The model under review builds one solid part; all positions refer to its coordinate system, in mm. A direction names the side the tool comes from. Coordinates: 2 decimals unless noted, no trailing zeros. Loops run counter-clockwise (first coordinate to the right, second up) from the corner with the lowest first, then second, coordinate; pieces in that order, holes last. Notation, with made-up numbers: M -39,13.5 L -30,13.5 A10 ccw -30,29.5 Z; hole C 13.5,83.25 d3. An arc over 180 degrees is marked long. Use one line per item in the form item = value.
Autodesk Inventor part; units mm, degrees
ref_plane "YZ Plane" through (0, 0, 0) normal (1, 0, 0) x (0, 1, 0)
ref_plane "XZ Plane" through (0, 0, 0) normal (0, 1, 0) x (-1, 0, 0)
ref_plane "XY Plane" through (0, 0, 0) normal (0, 0, 1) x (1, 0, 0)
sketch "Sketch1" plane through (0, 0, 0) normal (0, 0, 1) x (1, 0, 0)
  circle A0 centre (0, 0) radius 6.5
  dimension "d0" = 13
extrude "Extrusion1" add sketch "Sketch1" along normal blind 10
sketch "Sketch2" plane through (0, 0, 10) normal (0, 0, 1) x (1, 0, 0)
  circle A0 centre (0, 0) radius 5.5
  dimension "d3" = 11
extrude "Extrusion2" cut sketch "Sketch2" against normal blind 8
sketch "Sketch3" plane through (0, 0, 10) normal (0, 0, 1) x (1, 0, 0)
  circle A0 centre (0, 0) radius 5.5
  circle A1 centre (0, 0) radius 6.5
  line L0 (-2, 0) -> (2, 0)
  line L1 (2, 0) -> (2, -6.9117)
  line L2 (2, -6.9117) -> (-2, -6.9117)
  line L3 (-2, -6.9117) -> (-2, 0)
  dimension "d6" = 4
extrude "Extrusion3" cut sketch "Sketch3" against normal blind 4 contours L3 L0 L1 A0 | A0 L1 A1 L3 | A1 L1 L2 L3 picked at (0.2269, -1.8192) picked at (-1.5602, -5.5886)
properties part number "capuchon.torre"
1. Add section C-C (y = 0.25). State the section outline as (x, z) points.
Response values:
outline = M -6.5,0 L 6.5,0 L 6.5,10 L 5.49,10 L 5.49,2 L -5.49,2 L -5.49,10 L -6.5,10 Z
2. Add section A-A (x = 0). State the section outline as (y, z) points, then the cut area to 3 significant figures.
Response values:
outline = M -6.5,0 L 6.5,0 L 6.5,10 L 5.5,10 L 5.5,2 L -5.5,2 L -5.5,6 L -6.5,6 Z
area = 38.0 mm^2
3. Machinability: for faces 1 (the face through (0, 0, 0)), 2 (the face through (-2, -6, 8)), which of the approach directions +Z, -Z, +X, -X, +Y, -Y give a long, thin tool a straight path to every point of the face, cutting with its end or side? Answer none if there is none.
Response values:
face_1 = -Z, +X, -X, +Y, -Y
face_2 = +Z, -Y
4. Insertion check: P1, Ø0.8, axis at y = -6, z = 7, coming from the +X side; P2, Ø1.5, axis at x = -3.5, y = 0.5, coming from the +Z side; P3, Ø3, axis at y = 3.5, z = 8, coming from the -X side. Each pin has a flat end and moves straight along its axis. Give the tip position at first contact, or say it passes through.
Response values:
P1 = 3.3
P2 = 2
P3 = -6.18
5. The part is to be moulded in two halves that separate along Y. For faces 3 (the face through (0, 0, 2)), 4 (the face through (-0.716, 5.453, 6.056)), 5 (the face through (-1.409, 6.345, 4.93)), 6 (the face through (-4, 4, 10)), say which applies: pulls with the +Y half, pulls with the -Y half, needs draft (parallel to the pull), parting line crosses it, or undercut.
Response values:
face_3 = undercut
face_4 = undercut
face_5 = parting line crosses it
face_6 = needs draft
6. Wall thickness on line 1 along X through (y, z) = (0, 4); line 2 along Z through (x, y) = (0.25, 3): over which ranges is each line inside the solid? List them lowest first. Write a range as from..to.
Response values:
line_1 = -6.5..-5.5, 5.5..6.5
line_2 = 0..2
7. Add section B-B (z = 3.5). State the section outline as (x, y) points, then the cut area to 3 significant figures.
Response values:
outline = C 0,0 d13; hole C 0,0 d11
area = 37.7 mm^2
8. Add section D-D (z = 9). State the section outline as (x, y) points, then the cut area to 3 significant figures.
Response values:
outline = M -2,-6.18 L -2,-5.12 A5.5 cw long 2,-5.12 L 2,-6.18 A6.5 ccw long Z
area = 33.6 mm^2
